```python
from build123d import *

# Parameters (mm, degrees)
SKETCH1_W            = 120
SKETCH1_H            = 110
BOSS_EXTRUDE1_DEPTH  = 6
SKETCH2_R            = 33.55
CUT_EXTRUDE1_DEPTH   = 82.614949611
M3_CLEARANCE_HOLE1_D = 3.1
CIRPATTERN1_COUNT    = 12
M6_CLEARANCE_HOLE2_D = 6.1


with BuildPart() as part:
    # Sketch1 → Boss-Extrude1 (new body)
    with BuildSketch(Plane(origin=(0, 0, 0), x_dir=(1, 0, 0), z_dir=(0, 1, 0))):
        Rectangle(SKETCH1_W, SKETCH1_H)
    extrude(amount=BOSS_EXTRUDE1_DEPTH)

    # Sketch2 → Cut-Extrude1 (cut, through all)
    with BuildSketch(Plane(origin=(0, 6, 0), x_dir=(1, 0, 0), z_dir=(0, 1, 0))):
        with Locations(Location((0, 0, 0), (0, 0, 270))):
            Circle(SKETCH2_R)
    extrude(amount=-CUT_EXTRUDE1_DEPTH, mode=Mode.SUBTRACT)

    # M3 Clearance Hole1 (through all)
    with Locations(Plane(origin=(0, 6, 0), x_dir=(1, 0, 0), z_dir=(0, 1, 0))):
        with Locations((0, 37)):
            m3_clearance_hole1 = Hole(M3_CLEARANCE_HOLE1_D / 2)

    # CirPattern1: M3 Clearance Hole1 ×12 about axis
    cirpattern1_axis = Axis((0, 0, 0), (0, 1, 0))
    for i in range(1, CIRPATTERN1_COUNT):
        add(m3_clearance_hole1.rotate(cirpattern1_axis, i * 360 / CIRPATTERN1_COUNT), mode=Mode.SUBTRACT)

    # M6 Clearance Hole2 (through all)
    with Locations(Plane(origin=(0, 6, 0), x_dir=(1, 0, 0), z_dir=(0, 1, 0))):
        with Locations((52.5, -45), (52.5, -15), (52.5, 15), (52.5, 45)):
            m6_clearance_hole2 = Hole(M6_CLEARANCE_HOLE2_D / 2)

    # Mirror1: M6 Clearance Hole2 across plane
    add(m6_clearance_hole2.mirror(Plane(origin=(0, 0, 0), x_dir=(0, 0, 1), z_dir=(1, 0, 0))), mode=Mode.SUBTRACT)


solid = part.part
```
Work out the finished part from the listing and answer in its coordinate system (mm). Coordinates: 2 decimals unless noted, no trailing zeros. Write each loop counter-clockwise with the first axis right and the second up, starting at its lowest first coordinate (ties: lowest second). Pieces come first, ordered by that corner, then holes. Notation, with made-up numbers: (-9, 59.5) - (14, 59.5) arc R12 cw to (14, 66.5) - close; hole circle Ø2 at (4.5, 43). An arc over 180 degrees is marked (long way). Answer as a JSON object with one key per item and string values.
Q1. Given pin 1 Ø8 at (x, z) = (52.5, -45) entering from -Y, flat-ended and moving along its own axis, determine where the tip first touches the part or whether it passes through.
Results list:
{"pin 1": "stops at y = 0"}
Q2. Find section C-C (z = 37). Write down the section's boundary in (x, y).
Results list:
{"outline": "(-60, 0) - (-1.55, 0) - (-1.55, 6) - (-60, 6) - close; (1.55, 0) - (60, 0) - (60, 6) - (1.55, 6) - close"}
Q3. Consider L1, parallel to Z at x = -52.5, y = 3.1; L2, parallel to X at y = 2.8, z = -18.5; L3, parallel to X at y = 1.25, z = 0. Determine where each line is inside the solid, lowest interval first. Write a range as from..to.
Results list:
{"L1": "z = -55..-48.05, -41.95..-18.05, -11.95..11.95, 18.05..41.95, 48.05..55", "L2": "x = -60..-33.59, -30.49..-27.99, 27.99..30.49, 33.59..60", "L3": "x = -60..-38.55, -35.45..-33.55, 33.55..35.45, 38.55..60"}
Q4. For a pull along Z with two mould halves and no side action, classify faces 1 (the flat face through (-28, 6, 24)), 2 (the cylindrical face through (-20.415, 3.042, -26.624)) as pulls with the +Z half, pulls with the -Z half, needs draft (parallel to the pull), parting line crosses it, or undercut.
Results list:
{"face 1": "needs draft", "face 2": "undercut"}
Q5. Find section B-B (z = 0). Write down the section's boundary in (x, y).
Results list:
{"outline": "(-60, 0) - (-38.55, 0) - (-38.55, 6) - (-60, 6) - close; (-35.45, 0) - (-33.55, 0) - (-33.55, 6) - (-35.45, 6) - close; (33.55, 0) - (35.45, 0) - (35.45, 6) - (33.55, 6) - close; (38.55, 0) - (60, 0) - (60, 6) - (38.55, 6) - close"}
Q6. Find section D-D (x = 52.5). Write down the section's boundary in (y, z).
Results list:
{"outline": "(0, -55) - (6, -55) - (6, -48.05) - (0, -48.05) - close; (0, -41.95) - (6, -41.95) - (6, -18.05) - (0, -18.05) - close; (0, -11.95) - (6, -11.95) - (6, 11.95) - (0, 11.95) - close; (0, 18.05) - (6, 18.05) - (6, 41.95) - (0, 41.95) - close; (0, 48.05) - (6, 48.05) - (6, 55) - (0, 55) - close"}
Q7. Find section A-A (x = 37). Write down the section's boundary in (y, z).
Results list:
{"outline": "(0, -55) - (6, -55) - (6, -1.55) - (0, -1.55) - close; (0, 1.55) - (6, 1.55) - (6, 55) - (0, 55) - close"}
